Read the model definition and answer for the solid it produces. Units are mm, in the model's axes. A direction names the side the tool comes from. Round coordinates to 2 decimals unless told otherwise and drop trailing zeros. Loops run counter-clockwise (first coordinate to the right, second up) from the corner with the lowest first, then second, coordinate; pieces in that order, holes last. Notation, with made-up numbers: (30, 34) -> (72, 34) arc R19 cw to (72, 60) -> close; hole circle Ø6 at (-35, 66.25). An arc over 180 degrees is marked (long way). Put each result on its own line as item: value.
from build123d import *

# Parameters (mm, degrees)
F1_DEPTH = 2130
F2_R     = 5.08
F3_R     = 5.08


with BuildPart() as f1:
    # F0 (on Front) → F1 (new body)
    with BuildSketch(Plane.XZ):
        Polygon((48.768, 76.2), (0, 76.2), (0, 0), (5.08, 0), (5.08, 67.4878), (48.768, 67.4878), align=None)
        Polygon((5.08, 0), (0, 0), (0, -76.2), (48.768, -76.2), (48.768, -67.4878), (5.08, -67.4878), align=None)
    extrude(amount=F1_DEPTH)

    # F2
    f2_edges = [f1.edges().sort_by_distance(p)[0] for p in [
        (5.08, -1065, -67.4878),
        (5.08, -1065, 67.4878),
    ]]
    fillet(f2_edges, radius=F2_R)

    # F3
    f3_edges = [f1.edges().sort_by_distance(p)[0] for p in [
        (48.768, -1065, 67.4878),
        (48.768, -1065, -67.4878),
    ]]
    fillet(f3_edges, radius=F3_R)


solid = f1.part
Item 1: For a pull along Z with two mould halves and no side action, classify faces 3 (the flat face through (27, -1050, -67.488)), 4 (the flat face through (24, -1050, -76.2)), 5 (the flat face through (4, -2130, 6)), 6 (the flat face through (5.08, -1050, -1)) as pulls with the +Z half, pulls with the -Z half, needs draft (parallel to the pull), parting line crosses it, or undercut.
Derived:
face 3: undercut
face 4: pulls with the -Z half
face 5: needs draft
face 6: undercut
Item 2: Find the intervals of material crossed by line 1 along Z through (x, y) = (25, -1482); line 2 along Z through (x, y) = (9, -127); line 3 along X through (y, z) = (-553, 55.5), in increasing order.
Derived:
line 1: z = -76.2 to -67.49, 67.49 to 76.2
line 2: z = -76.2 to -67.35, 67.35 to 76.2
line 3: x = 0 to 5.08
Item 3: The part is cut by section C-C (z = -20.5). Determine the outline of the cut face in (x, y).
Derived:
outline: (0, -2130) -> (5.08, -2130) -> (5.08, 0) -> (0, 0) -> close
Item 4: The part is cut by section A-A (y = -1727.5). Determine the outline of the cut face in (x, z).
Derived:
outline: (0, -76.2) -> (48.77, -76.2) -> (48.77, -72.57) arc R5.08 ccw to (43.69, -67.49) -> (10.16, -67.49) arc R5.08 cw to (5.08, -62.41) -> (5.08, 62.41) arc R5.08 cw to (10.16, 67.49) -> (43.69, 67.49) arc R5.08 ccw to (48.77, 72.57) -> (48.77, 76.2) -> (0, 76.2) -> close
Item 5: Which of the six approach directions +Z, -Z, +X, -X, +Y, -Y give full straight-line access (tool end or side, diameter ignored) to faces 1 (the flat face through (4, 0, 6)), 2 (the flat face through (27, -1050, 67.488))?
Derived:
face 1: +Z, -Z, +X, -X, +Y
face 2: +X, +Y, -Y
Item 6: The part is cut by section B-B (x = 30). Determine the outline of the cut face in (y, z).
Derived:
outline: (-2130, -76.2) -> (0, -76.2) -> (0, -67.49) -> (-2130, -67.49) -> close; (-2130, 67.49) -> (0, 67.49) -> (0, 76.2) -> (-2130, 76.2) -> close
